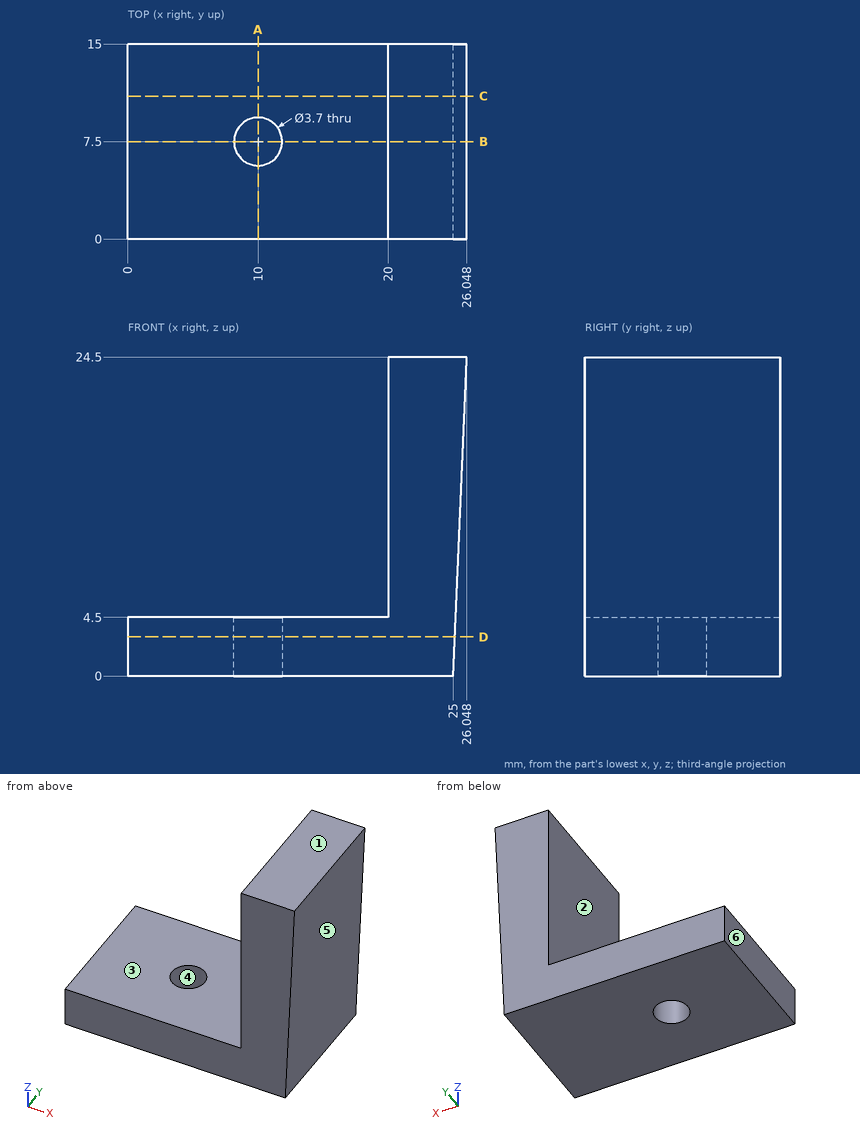
Verification items for this drawing (mm, ordinates from the low corner). A direction names the side the tool comes from. Round coordinates to 2 decimals unless told otherwise and drop trailing zeros. Order: outer loops, then holes, each group sorted by start corner. A loop starts at its lowest first (then second) coordinate and runs counter-clockwise, first axis right, second up. Notation, with made-up numbers: (-23.5, 45) -> (-6.5, 45) arc R32 ccw to (-6.5, 81) -> close; hole circle Ø6 at (-25.75, 77). An arc over 180 degrees is marked (long way). Use one line per item in the form item = value.
1. Scan lines: line 1 along Y through (x, z) = (10, 2.8); line 2 along Z through (x, y) = (8.5, 9); line 3 along X through (y, z) = (12.5, 6). Record each from-to range of solid material in increasing order. Write a range as from..to.
Working result:
line_1 = 0..5.65, 9.35..15
line_2 = 0..4.5
line_3 = 20..25.26
2. Cross-section at A-A, the plane x = 10. Enter the section's corners in (y, z).
Working result:
outline = (0, 0) -> (5.65, 0) -> (5.65, 4.5) -> (0, 4.5) -> close; (9.35, 0) -> (15, 0) -> (15, 4.5) -> (9.35, 4.5) -> close
3. Cross-section at C-C, the plane y = 11. Enter the section's corners in (x, z), plus the area to 3 significant figures.
Working result:
outline = (0, 0) -> (25, 0) -> (26.05, 24.5) -> (20, 24.5) -> (20, 4.5) -> (0, 4.5) -> close
area = 225 mm^2
4. Cross-section at D-D, the plane z = 3. Enter the section's corners in (x, y), plus the area to 3 significant figures.
Working result:
outline = (0, 0) -> (25.13, 0) -> (25.13, 15) -> (0, 15) -> close; hole circle Ø3.7 at (10, 7.5)
area = 366 mm^2
5. Go/stop test with flat-tipped pins: pin 1 (5 mm diameter, centred on y = 7.5, z = 15, fed in from +X); pin 2 (4 mm diameter, centred on y = 9.5, z = 21.5, fed in from -X); pin 3 (2 mm diameter, centred on y = 2, z = 7, fed in from +X). Record where each tip stops, or that it passes through.
Working result:
pin_1 = 25.75
pin_2 = 20
pin_3 = 25.34
6. Mould release check, pull along X, two halves, no side actions. Record for the marked faces 3, 4, 5 and 6: pulls with the +X half, pulls with the -X half, needs draft (parallel to the pull), parting line crosses it, or undercut.
Working result:
face_3 = needs draft
face_4 = undercut
face_5 = pulls with the +X half
face_6 = pulls with the -X half
7. Cross-section at B-B, the plane y = 7.5. Enter the section's corners in (x, z).
Working result:
outline = (0, 0) -> (8.15, 0) -> (8.15, 4.5) -> (0, 4.5) -> close; (11.85, 0) -> (25, 0) -> (26.05, 24.5) -> (20, 24.5) -> (20, 4.5) -> (11.85, 4.5) -> close
8. Set-up check for the marked faces 1 and 2: record each of +Z, -Z, +X, -X, +Y, -Y from which the full face is reachable in a straight line by a thin tool's end or side.
Working result:
face_1 = +Z, +X, -X, +Y, -Y
face_2 = +Z, -X, +Y, -Y
